Check sheet for the modelled part. Datum: model origin and axes. Units: mm. Give positions to 0.01 mm unless a question says otherwise; leave off trailing zeros. Loops run counter-clockwise (first coordinate to the right, second up) from the corner with the lowest first, then second, coordinate; pieces in that order, holes last. Notation, with made-up numbers: M 21,62.25 L 72,62.25 A23 ccw 72,99.25 Z; hole C 73.25,10.25 d8. An arc over 180 degrees is marked long. Write each question's results on one line, items separated by ' | '. Start each with the question number.
1. Material ranges on line 1 along X through (y, z) = (7.5, -6.5) (3 decimals); line 2 along X through (y, z) = (-5, -8.25) (3 decimals); line 3 along Z through (x, y) = (21.5, -0.5), recorded low to high.
2. Go/stop test with flat-tipped pins: pin 1 (3 mm diameter, centred on x = 2, z = -8, fed in from -Y); pin 2 (5 mm diameter, centred on x = -14.5, y = 7.5, fed in from +Z). Record where each tip stops, or that it passes through.
3. Sectioned sample at A-A on x = 22.5. Record the cut outline in (y, z), and give its area (3 significant figures).
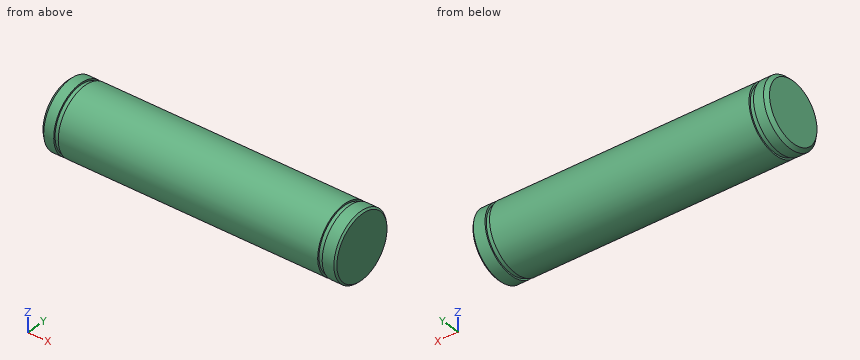
```python
from build123d import *

# Parameters (mm, degrees)
SKETCH1_R           = 10
BOSS_EXTRUDE1_DEPTH = 44.175
SKETCH2_R           = 10
SKETCH2_R_2         = 9.5
CUT_EXTRUDE1_DEPTH  = 1.35
CHAMFER1_SIZE       = 0.5
CHAMFER2_SIZE       = 1


with BuildPart() as part:
    # Sketch1 → Boss-Extrude1 (new, symmetric)
    with BuildSketch(Plane(origin=(0, 0, 0), x_dir=(0, 0, -1), z_dir=(1, 0, 0))):
        Circle(SKETCH1_R)
    extrude(amount=BOSS_EXTRUDE1_DEPTH, both=True)

    # Sketch2 → Cut-Extrude1 (cut)
    with BuildSketch(Plane(origin=(40.175, 0, 0), x_dir=(0, 0, -1), z_dir=(1, 0, 0))):
        Circle(SKETCH2_R)
        Circle(SKETCH2_R_2, mode=Mode.SUBTRACT)
    cut_extrude1 = extrude(amount=-CUT_EXTRUDE1_DEPTH, mode=Mode.SUBTRACT)

    # Chamfer1
    chamfer1_edges = [part.edges().sort_by_distance(p)[0] for p in [
        (44.175, 0, 10),
    ]]
    chamfer(chamfer1_edges, length=CHAMFER1_SIZE)

    # Chamfer2
    chamfer2_edges = [part.edges().sort_by_distance(p)[0] for p in [
        (-44.175, 0, 10),
    ]]
    chamfer(chamfer2_edges, length=CHAMFER2_SIZE)

    # Mirror1: Cut-Extrude1 across plane
    add(cut_extrude1.mirror(Plane(origin=(0, 0, 0), x_dir=(0, 0, 1), z_dir=(1, 0, 0))), mode=Mode.SUBTRACT)


solid = part.part
```
Output values:
1) line 1: -43.25 to -40.175, -38.825 to 38.825, 40.175 to 43.75 | line 2: -43.528 to -40.175, -38.825 to 38.825, 40.175 to 44.028 | line 3: -9.99 to 9.99
2) pin 1: y = -7.6 | pin 2: z = 8.66
3) outline: C 0,0 d20 | area: 314 mm2
